```python
from build123d import *

# Parameters (mm, degrees)
F0_R     = 36.75
F1_DEPTH = 1
F2_R     = 33.75
F2_W     = 1.7
F2_H     = 3
F3_DEPTH = 0.5
F4_DEPTH = 2


with BuildPart() as f1:
    # F0 (on Top) → F1 (new body)
    with BuildSketch(Plane.XY):
        Circle(F0_R)
    extrude(amount=F1_DEPTH)

    # F2 (on face) → F3 (join)
    with BuildSketch(Plane.XY.offset(1)):
        Circle(F2_R)
        with Locations((0, -31.85)):
            Rectangle(F2_W, F2_H, mode=Mode.SUBTRACT)
        with Locations((0, 31.85)):
            Rectangle(F2_W, F2_H, mode=Mode.SUBTRACT)
    extrude(amount=F3_DEPTH)

    # F4 (add): faces of the model
    f4_faces = [f1.faces().sort_by_distance(p)[0] for p in [
        (0, -31.85, 1),
        (0, 31.85, 1),
    ]]
    extrude(f4_faces, amount=F4_DEPTH)


solid = f1.part
```
Build history of the part. All positions in model axes, mm. A direction names the side the tool comes from. Coordinates: 2 decimals unless noted, no trailing zeros. Order: outer loops, then holes, each group sorted by start corner. A loop starts at its lowest first (then second) coordinate and runs counter-clockwise, first axis right, second up. Notation, with made-up numbers: (-1.5, 34.5) -> (17.5, 34.5) arc R25 cw to (17.5, 46.5) -> close; hole circle Ø2 at (65, 40). An arc over 180 degrees is marked (long way). Answer in a Markdown table with one row per item. Add a question column.
Q1. Band-saw the part on B-B, the plane x = 0. List the corners of the cut face in (y, z), then the cut area to 3 significant figures.
Q2. Which spindle directions (+Z, -Z, +X, -X, +Y, -Y) get a long thin tool onto all of the face, cutting with end or side? Do faces 1 (the face through (0, -32, 3)), 2 (the face through (16, -30, 1)). Say none if no direction does.
Q3. Band-saw the part on D-D, the plane x = -14. List the corners of the cut face in (y, z).
Q4. Wall check: line 1 along Z through (x, y) = (-7.5, -33); line 2 along Z through (x, y) = (24, 14); line 3 along X through (y, z) = (29.5, 0.2). Give the ranges that are in metal, low to high. Write a range as [from, to].
Q5. Band-saw the part on C-C, the plane y = 0. List the corners of the cut face in (x, z).
Q6. Band-saw the part on A-A, the plane z = 2.4. List the corners of the cut face in (x, y), then the cut area to 3 significant figures.
Q7. Drop flat-ended pins along their axis: pin 1 (1.2 mm diameter, centred on y = -32.5, z = 2.5, fed in from +X); pin 2 (1.6 mm diameter, centred on x = -0.5, z = 2.5, fed in from -Y); pin 3 (3 mm diameter, centred on x = -19, y = 5.5, fed in from +Z). Give the stop position or say it passes through.
Answers follow:
| question | item | result |
|---|---|---|
| 1 | outline | (-36.75, 0) -> (36.75, 0) -> (36.75, 1) -> (33.75, 1) -> (33.75, 1.5) -> (33.35, 1.5) -> (33.35, 3) -> (30.35, 3) -> (30.35, 1.5) -> (-30.35, 1.5) -> (-30.35, 3) -> (-33.35, 3) -> (-33.35, 1.5) -> (-33.75, 1.5) -> (-33.75, 1) -> (-36.75, 1) -> close |
| 1 | area | 116 mm^2 |
| 2 | face 1 | +Z, +X, -X, +Y, -Y |
| 2 | face 2 | +Z |
| 3 | outline | (-33.98, 0) -> (33.98, 0) -> (33.98, 1) -> (30.71, 1) -> (30.71, 1.5) -> (-30.71, 1.5) -> (-30.71, 1) -> (-33.98, 1) -> close |
| 4 | line 1 | [0, 1] |
| 4 | line 2 | [0, 1.5] |
| 4 | line 3 | [-21.92, 21.92] |
| 5 | outline | (-36.75, 0) -> (36.75, 0) -> (36.75, 1) -> (33.75, 1) -> (33.75, 1.5) -> (-33.75, 1.5) -> (-33.75, 1) -> (-36.75, 1) -> close |
| 6 | outline | (-0.85, -33.35) -> (0.85, -33.35) -> (0.85, -30.35) -> (-0.85, -30.35) -> close; (-0.85, 30.35) -> (0.85, 30.35) -> (0.85, 33.35) -> (-0.85, 33.35) -> close |
| 6 | area | 10.2 mm^2 |
| 7 | pin 1 | x = 0.85 |
| 7 | pin 2 | y = -33.35 |
| 7 | pin 3 | z = 1.5 |
